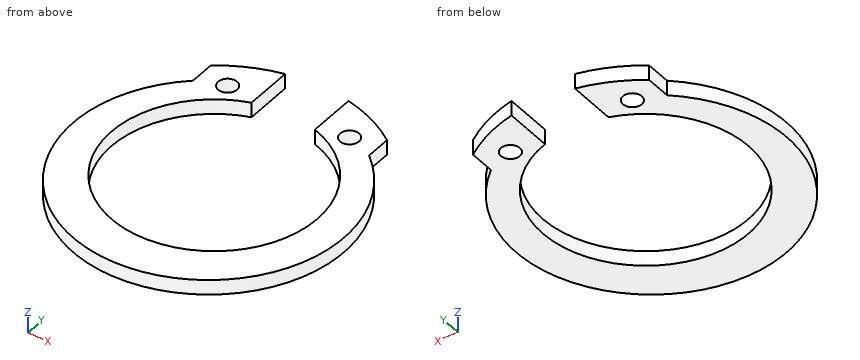
```python
from build123d import *

# Parameters (mm, degrees)
BOSS_EXTRUDE1_DEPTH            = 0.55
SKETCH2_R                      = 3.8
CUT_EXTRUDE1_DEPTH             = 1.55
CUT_EXTRUDE2_DEPTH             = 1.55
F_0_7_0_7_DIAMETER_HOLE1_D     = 0.7
F_0_7_0_7_DIAMETER_HOLE1_DEPTH = 0.55


with BuildPart() as part:
    # Sketch1 → Boss-Extrude1 (new body)
    with BuildSketch(Plane.XY):
        with BuildLine():
            Line((-3.25, 4.737059837), (-3.25, 3.799671038))
            ThreePointArc((-3.25, 3.799671038), (0, -5), (3.25, 3.799671038))
            Line((3.25, 3.799671038), (3.25, 4.737059837))
            ThreePointArc((3.25, 4.737059837), (0, 5.8), (-3.25, 4.737059837))
        make_face()
    extrude(amount=-BOSS_EXTRUDE1_DEPTH)

    # Sketch2 → Cut-Extrude1 (cut, through all)
    with BuildSketch(Plane.XY):
        with Locations((0, 0.3)):
            Circle(SKETCH2_R)
    extrude(amount=-CUT_EXTRUDE1_DEPTH, mode=Mode.SUBTRACT)

    # Sketch3 → Cut-Extrude2 (cut, through all)
    with BuildSketch(Plane.XY):
        with BuildLine():
            Line((-1.17, 5.67411388), (-1.17, 3.915397627))
            ThreePointArc((-1.17, 3.915397627), (0, 4.1), (1.17, 3.915397627))
            Line((1.17, 3.915397627), (1.17, 5.67411388))
            ThreePointArc((1.17, 5.67411388), (0, 5.8), (-1.17, 5.67411388))
        make_face()
    extrude(amount=-CUT_EXTRUDE2_DEPTH, mode=Mode.SUBTRACT)

    # Ø0.7 (0.7) Diameter Hole1
    with Locations(Plane.XY):
        with Locations((-2.25, 4.197114317), (2.25, 4.197114317)):
            Hole(F_0_7_0_7_DIAMETER_HOLE1_D / 2, depth=F_0_7_0_7_DIAMETER_HOLE1_DEPTH)


solid = part.part
```
For this review, take the finished solid that the model builds, in its own axes (mm). Coordinates: 2 decimals unless noted, no trailing zeros. Loops run counter-clockwise (first coordinate to the right, second up) from the corner with the lowest first, then second, coordinate; pieces in that order, holes last. Notation, with made-up numbers: (-26.5, 85.5) -> (5.5, 85.5) arc R16 cw to (5.5, 94.5) -> close; hole circle Ø3 at (-5.5, -15). An arc over 180 degrees is marked (long way). Return JSON: item names as keys, results as strings. Group by question number.
(1) For pin 1 Ø3 at (x, y) = (1.5, -0.5) entering from -Z, flat-tipped, find the tip position at first contact; note if it passes through.
(2) Consider section D-D, the plane x = 0. Give the boundary of the cut face in (y, z).
(3) To check wall thickness, follow L1, parallel to Y at x = 2.25, z = -0.1; L2, parallel to X at y = -2.25, z = -0.05; L3, parallel to Y at x = 0, z = -0.3. State the ranges of each line that lie inside material, in increasing order.
(4) Consider section C-C, the plane x = 2.25. Give the boundary of the cut face in (y, z), plus the area to 3 significant figures.
(5) Consider section A-A, the plane y = 1. Give the boundary of the cut face in (x, z), plus the area to 3 significant figures.
(6) Consider section B-B, the plane x = 3.5. Give the boundary of the cut face in (y, z).
Results below:
{
 "1": {"pin 1": "passes through"},
 "2": {"outline": "(-5, -0.55) -> (-3.5, -0.55) -> (-3.5, 0) -> (-5, 0) -> close"},
 "3": {"L1": "y = -4.47 to -2.76, 3.36 to 3.85, 4.55 to 5.32", "L2": "x = -4.47 to -2.82, 2.82 to 4.47", "L3": "y = -5 to -3.5"},
 "4": {"outline": "(-4.47, -0.55) -> (-2.76, -0.55) -> (-2.76, 0) -> (-4.47, 0) -> close; (3.36, -0.55) -> (3.85, -0.55) -> (3.85, 0) -> (3.36, 0) -> close; (4.55, -0.55) -> (5.32, -0.55) -> (5.32, 0) -> (4.55, 0) -> close", "area": "1.63 mm2"},
 "5": {"outline": "(-4.9, -0.55) -> (-3.73, -0.55) -> (-3.73, 0) -> (-4.9, 0) -> close; (3.73, -0.55) -> (4.9, -0.55) -> (4.9, 0) -> (3.73, 0) -> close", "area": "1.28 mm2"},
 "6": {"outline": "(-3.57, -0.55) -> (-1.18, -0.55) -> (-1.18, 0) -> (-3.57, 0) -> close; (1.78, -0.55) -> (3.57, -0.55) -> (3.57, 0) -> (1.78, 0) -> close"}
}
